Source: three-view drawing plus pictorial views. Frame: mm from the lowest corner of the part. Coordinates: 2 decimals unless noted, no trailing zeros. Loops run counter-clockwise (first coordinate to the right, second up) from the corner with the lowest first, then second, coordinate; pieces in that order, holes last. Notation, with made-up numbers: M -13.5,-27.75 L 14.5,-27.75 A15 ccw 14.5,-23.75 Z; hole C 76,-12.75 d11. An arc over 180 degrees is marked long. Use a Markdown table: item, result. Add a question column.
1. Pin query (flat end, axial travel): pin 1 (3 mm diameter, centred on x = 34.5, z = 32.5, fed in from +Y); pin 2 (0.6 mm diameter, centred on y = 2.5, z = 11, fed in from +X); pin 3 (4 mm diameter, centred on x = 8, z = 8, fed in from +Y); pin 4 (1 mm diameter, centred on y = 2.5, z = 10, fed in from -X). Return the tip coordinate at first contact, or that it passes through.
2. Section A-A on x = 8. Output: boundary loops of the cut face in (y, z), then the cut area to 3 significant figures.
3. Line query: L1, parallel to Z at x = 36.5, y = 0.7; L2, parallel to Z at x = 22.7, y = 0.75; L3, parallel to X at y = 0.7, z = 8. Output: solid intervals per line, ascending. Write a range as [from, to].
4. Section C-C on y = 0.55. State how many separate pieces and enclosed holes the cut face has, then the cut area to 3 significant figures.
5. Section D-D on z = 27. Output: boundary loops of the cut face in (x, y).
6. Section B-B on z = 8.5. Output: boundary loops of the cut face in (x, y).
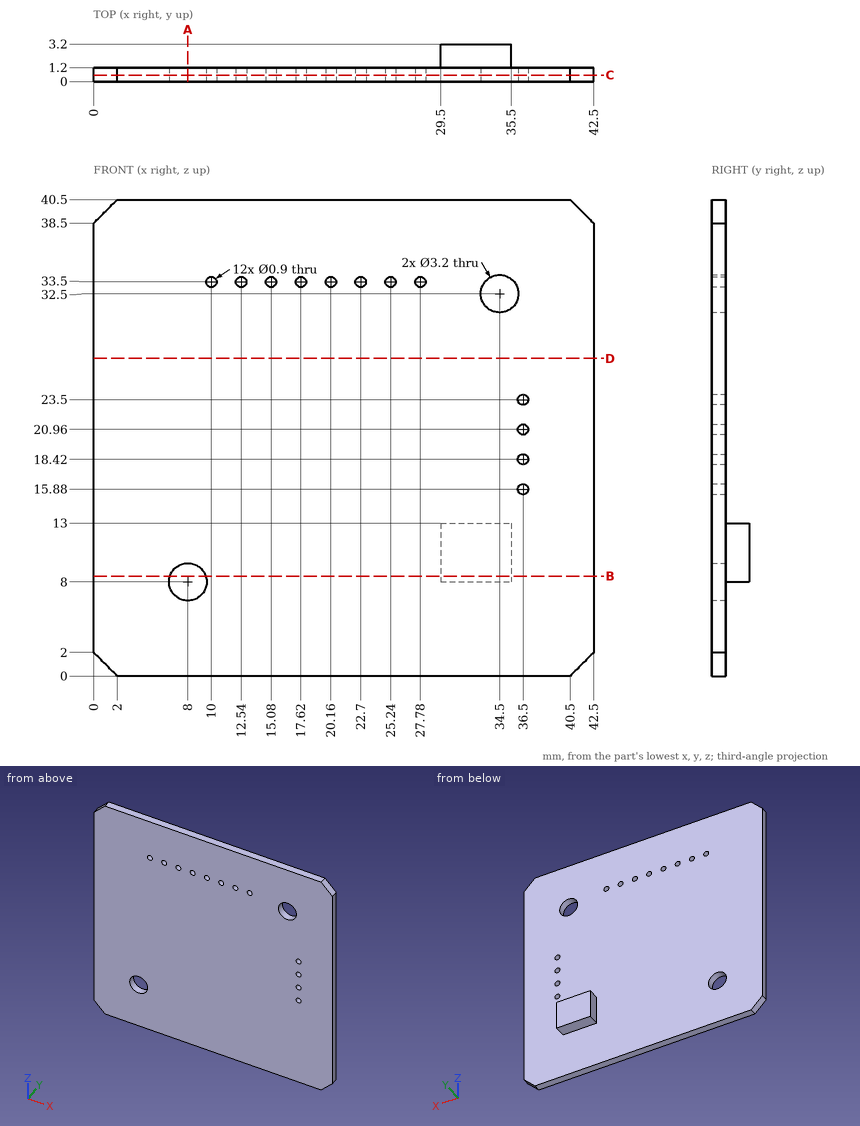
Answers below:
| question | item | result |
|---|---|---|
| 1 | pin 1 | passes through |
| 1 | pin 2 | stops at x = 35.5 |
| 1 | pin 3 | stops at y = 1.2 |
| 1 | pin 4 | stops at x = 29.5 |
| 2 | outline | M 0,0 L 1.2,0 L 1.2,6.4 L 0,6.4 Z; M 0,9.6 L 1.2,9.6 L 1.2,40.5 L 0,40.5 Z |
| 2 | area | 44.8 mm² |
| 3 | L1 | z = [0, 15.43], [16.33, 17.97], [18.87, 20.51], [21.41, 23.05], [23.95, 40.5] |
| 3 | L2 | z = [0, 33.05], [33.95, 40.5] |
| 3 | L3 | x = [0, 6.4], [9.6, 42.5] |
| 4 | separate pieces | 1 |
| 4 | enclosed holes | 14 |
| 4 | area | 1,690 mm² |
| 5 | outline | M 0,0 L 42.5,0 L 42.5,1.2 L 0,1.2 Z |
| 6 | outline | M 0,0 L 6.48,0 L 6.48,1.2 L 0,1.2 Z; M 9.52,0 L 42.5,0 L 42.5,1.2 L 35.5,1.2 L 35.5,3.2 L 29.5,3.2 L 29.5,1.2 L 9.52,1.2 Z |
